Check sheet for the modelled part. Datum: model origin and axes. Units: mm. Coordinates: 2 decimals unless noted, no trailing zeros. Write each loop counter-clockwise with the first axis right and the second up, starting at its lowest first coordinate (ties: lowest second). Pieces come first, ordered by that corner, then holes. Notation, with made-up numbers: M -30,-35.5 L 7,-35.5 A19 cw 7,0.5 Z; hole C 16,71 d5. An arc over 180 degrees is marked long. Answer as CSV lines item,"result". Start each with the question number.
1) Section check A-A (y = -3). Record the cut outline in (x, z).
2) Go/stop test with a flat-tipped pin: pin 1 Ø1.5 at (x, y) = (-1, -19.5) entering from -Z. Record where the tip stops, or that it passes through.
3) Section check B-B (x = 3.5). Record the cut outline in (y, z), and give its area (3 significant figures).
4) Section check C-C (z = -79.5). Record the cut outline in (x, y), and give its area (3 significant figures).
5) Material ranges on L1, parallel to Z at x = -70, y = -17.5; L2, parallel to X at y = -9, z = -86; L3, parallel to X at y = -17.25, z = -80.5, recorded low to high. Write a range as [from, to].
from build123d import *

# Parameters (mm, degrees)
F2_DEPTH = 25


with BuildPart() as f2:
    # F1 (on face) → F2 (new body)
    with BuildSketch(Plane.XZ):
        Polygon((19.5, 28.8766958117), (-90.7602548171, 28.8766958117), (-90.7602548171, -77.0238212563), (-69.3126782044, -96.7205752883), (-2.1988731881, -96.7205752883), (19.5, -73.0591952168), align=None)
    extrude(amount=F2_DEPTH)


solid = f2.part
Results found:
1,outline,"M -90.76,-77.02 L -69.31,-96.72 L -2.2,-96.72 L 19.5,-73.06 L 19.5,28.88 L -90.76,28.88 Z"
2,pin 1,"stops at z = -96.23"
3,outline,"M -25,-90.51 L 0,-90.51 L 0,28.88 L -25,28.88 Z"
3,area,"2,980 mm2"
4,outline,"M -88.06,-25 L 13.59,-25 L 13.59,0 L -88.06,0 Z"
4,area,"2,540 mm2"
5,L1,"z = [-96.09, 28.88]"
5,L2,"x = [-80.99, 7.63]"
5,L3,"x = [-86.98, 12.68]"
